Answer from the drawing. Dimensions are ordinates in mm from the lowest x, y and z of the part. Give positions to 0.01 mm unless a question says otherwise; leave off trailing zeros. Write each loop counter-clockwise with the first axis right and the second up, starting at its lowest first coordinate (ties: lowest second). Pieces come first, ordered by that corner, then holes.
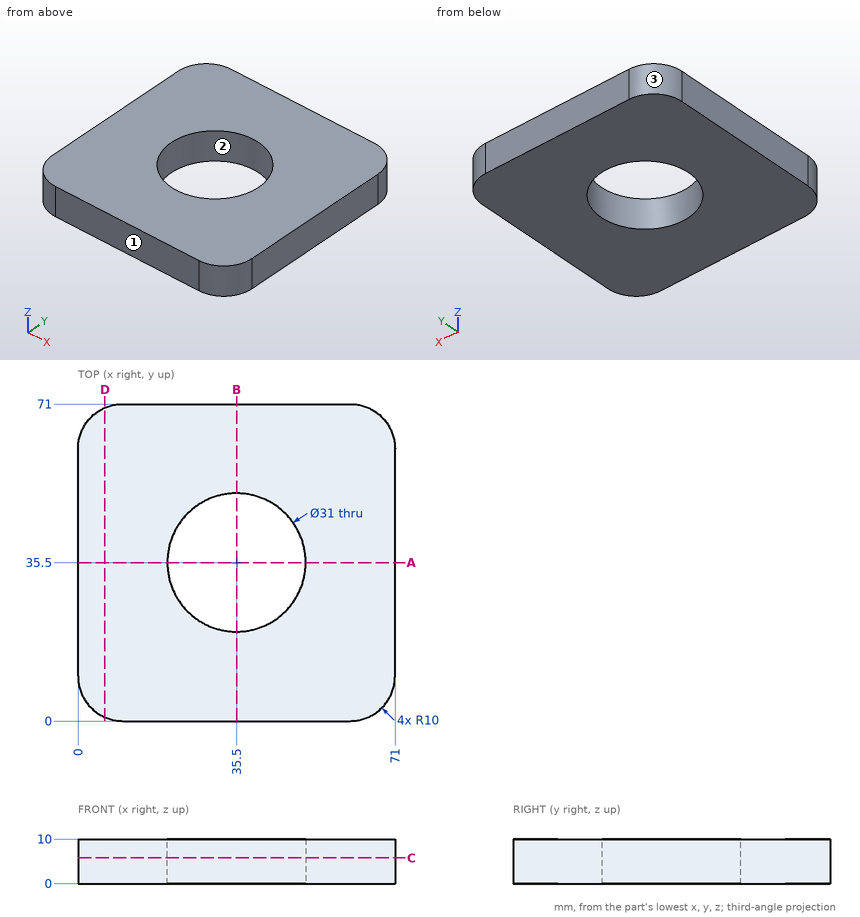
Item 1: Determine the mould class of the marked faces 1, 2 and 3 for opening direction Y: pulls with the +Y half, pulls with the -Y half, needs draft (parallel to the pull), parting line crosses it, or undercut.
Conclusion:
face 1: pulls with the -Y half
face 2: undercut
face 3: pulls with the +Y half
Item 2: Consider probe 1 along Y at (x, z) = (35.5, 4); probe 2 along Y at (x, z) = (25, 2.75); probe 3 along X at (y, z) = (29, 9.25). Determine where each line is inside the solid, lowest interval first.
Conclusion:
probe 1: y = 0 to 20, 51 to 71
probe 2: y = 0 to 24.1, 46.9 to 71
probe 3: x = 0 to 21.43, 49.57 to 71
Item 3: A cutting plane is placed at A-A, the plane y = 35.5. Give the vertices of the cut face in (x, z).
Conclusion:
outline: (0, 0) - (20, 0) - (20, 10) - (0, 10) - close; (51, 0) - (71, 0) - (71, 10) - (51, 10) - close
Item 4: This flat-tipped pin is pushed along its axis until it touches: P1, Ø1, axis at x = 9.5, z = 3, coming from the -Y side. Where does it stop, or does it pass through?
Conclusion:
P1: stops at y = 0
Item 5: A cutting plane is placed at C-C, the plane z = 5.75. Give the vertices of the cut face in (x, y).
Conclusion:
outline: (0, 10) arc R10 ccw to (10, 0) - (61, 0) arc R10 ccw to (71, 10) - (71, 61) arc R10 ccw to (61, 71) - (10, 71) arc R10 ccw to (0, 61) - close; hole circle Ø31 at (35.5, 35.5)
Item 6: A cutting plane is placed at D-D, the plane x = 6. Give the vertices of the cut face in (y, z), plus the area to 3 significant figures.
Conclusion:
outline: (0.83, 0) - (70.17, 0) - (70.17, 10) - (0.83, 10) - close
area: 693 mm2
